Can you work these out from the drawing? Everything is in mm from the part's minimum corner. A direction names the side the tool comes from. Give positions to 0.01 mm unless a question says otherwise; leave off trailing zeros. Loops run counter-clockwise (first coordinate to the right, second up) from the corner with the lowest first, then second, coordinate; pieces in that order, holes last. Notation, with made-up numbers: (77, 24.25) -> (87, 24.25) arc R24 cw to (87, 34.25) -> close; hole circle Ø8 at (38, 49). An arc over 180 degrees is marked (long way). Write item = value, one per line. Start each with the question number.
1) I want a section at B-B (z = 9). List the corners of the cut face in (x, y) for me (1 decimal).
2) I want a section at A-A (y = 2). List the corners of the cut face in (x, z) for me.
3) I need wall thicknesses on probe 1 along Y at (x, z) = (11, 8); probe 2 along Z at (x, y) = (6.5, 20.75); probe 3 along Z at (x, y) = (2.5, 1.75) (1 decimal). Which ranges of each line are inside material? Lowest first, please. Write a range as from..to.
4) On a 3-axis mill with a long thin cutter (end or side, diameter ignored), from which of +Z, -Z, +X, -X, +Y, -Y can I reach the whole of each face in a straight line? I mean the marked faces 1 and 2. Say none if no direction works.
5) I want a section at D-D (z = 10.5). List the corners of the cut face in (x, y) for me, and give its area (3 significant figures).
6) I want a section at C-C (y = 15.5). List the corners of the cut face in (x, z) for me (1 decimal).
7) I'm going to push flat-ended pins straight in: pin 1 Ø5 at (y, z) = (8, 6) entering from -X; pin 2 Ø5 at (y, z) = (5.5, 9) entering from -X; pin 3 Ø5 at (y, z) = (17.5, 3.5) entering from +X. Where does each tip first touch, or does it pass through?
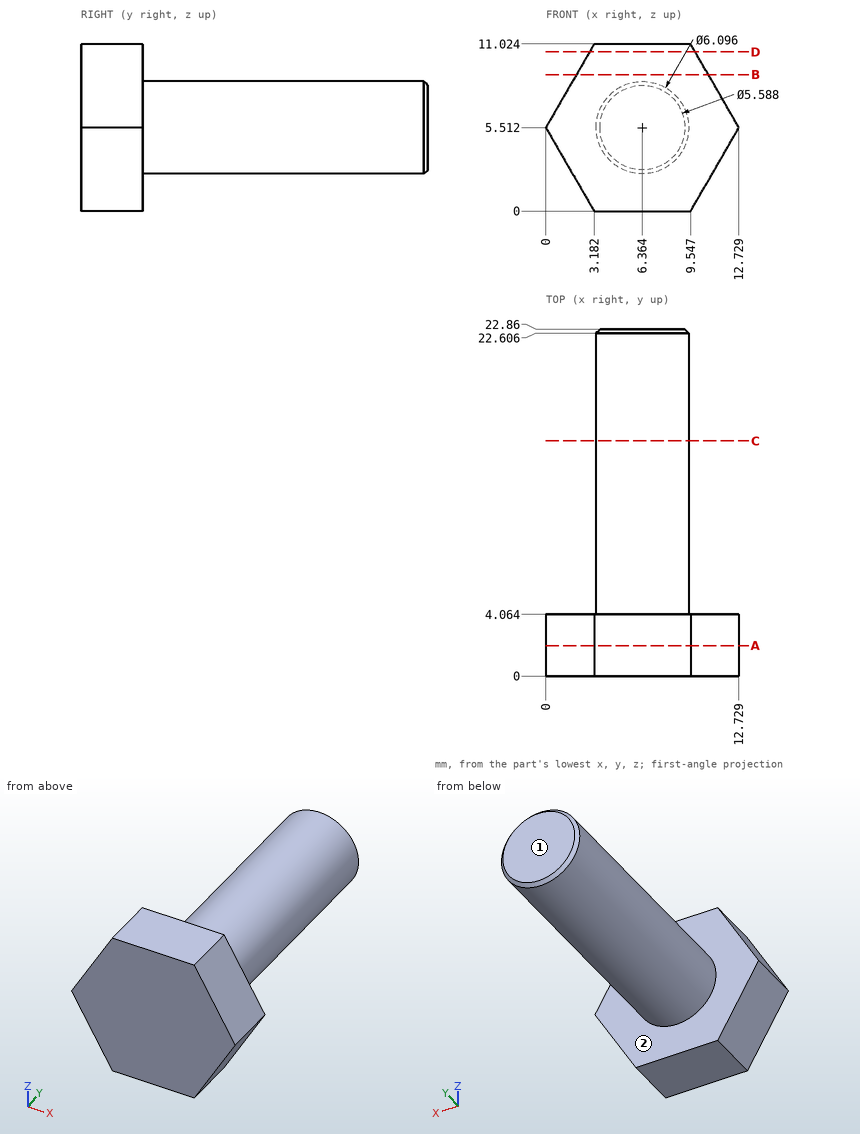
Answer list:
q1.outline = (2, 0) -> (10.7, 0) -> (10.7, 4.1) -> (2, 4.1) -> close
q2.outline = (0, 5.51) -> (3.18, 0) -> (9.55, 0) -> (12.73, 5.51) -> (9.55, 11.02) -> (3.18, 11.02) -> close
q3.probe_1 = 0..4.06
q3.probe_2 = 2.47..8.56
q3.probe_3 = 1.2..9.8
q4.face_1 = +Z, -Z, +X, -X, +Y
q4.face_2 = +Y
q5.outline = (2.88, 0) -> (9.85, 0) -> (9.85, 4.06) -> (2.88, 4.06) -> close
q5.area = 28.3 mm^2
q6.outline = circle Ø6.1 at (6.4, 5.5)
q7.pin_1 = 3.32
q7.pin_2 = 0.83
q7.pin_3 = 9.41
